Here's how the part is built. I have some questions about the finished solid (model axes, mm). Face numbers are marked on the shaded views. A direction names the side the tool comes from. Round coordinates to 2 decimals unless told otherwise and drop trailing zeros. Write each loop counter-clockwise with the first axis right and the second up, starting at its lowest first coordinate (ties: lowest second). Pieces come first, ordered by that corner, then holes. Notation, with made-up numbers: (-38.75, 59.5) - (-5.75, 59.5) arc R26 cw to (-5.75, 78.5) - close; hole circle Ø2 at (33.25, 30). An arc over 180 degrees is marked (long way). Return JSON: item names as keys, results as strings. Group by question number.
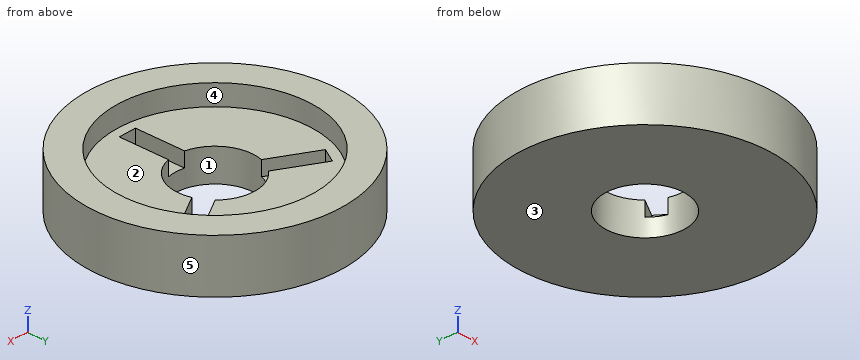
```python
from build123d import *

# Parameters (mm, degrees)
SKETCH_R           = 43.25
PAD_DEPTH          = 18
SKETCH001_R        = 33.25
POCKET_DEPTH       = 7
SKETCH002_R        = 13.5
POCKET001_DEPTH    = 11.001
SKETCH003_W        = 6
SKETCH003_H        = 30
POCKET002_DEPTH    = 5
POLARPATTERN_COUNT = 3


with BuildPart() as part:
    # Sketch → Pad (new body)
    with BuildSketch(Plane.XY):
        Circle(SKETCH_R)
    extrude(amount=PAD_DEPTH)

    # Sketch001 (on Face3 of Pad) → Pocket (cut)
    with BuildSketch(Plane.XY.offset(18)):
        Circle(SKETCH001_R)
    extrude(amount=-POCKET_DEPTH, mode=Mode.SUBTRACT)

    # Sketch002 (on Face5 of Pocket) → Pocket001 (cut, through all)
    with BuildSketch(Plane.XY.offset(11)):
        Circle(SKETCH002_R)
    extrude(amount=-POCKET001_DEPTH, mode=Mode.SUBTRACT)

    # Sketch003 (on Face6 of Pocket001) → Pocket002 (cut)
    with BuildSketch(Plane.XY.offset(11)):
        with Locations((0, -15)):
            Rectangle(SKETCH003_W, SKETCH003_H)
    pocket002 = extrude(amount=-POCKET002_DEPTH, mode=Mode.SUBTRACT)

    # PolarPattern: Pocket002 ×3 about axis
    polarpattern_axis = Axis((0, 0, 11), (0, 0, 1))
    for i in range(1, POLARPATTERN_COUNT):
        add(pocket002.rotate(polarpattern_axis, i * 360 / POLARPATTERN_COUNT), mode=Mode.SUBTRACT)


solid = part.part
```
1) Imagine slicing it at D-D (z = 4.5). Please give me the cut outline in (x, y), plus the area to 3 significant figures.
2) I need wall thicknesses on line 1 along Y through (x, z) = (0, 13.5); line 2 along Y through (x, z) = (0, 3.25); line 3 along X through (y, z) = (1.5, 14.75). Which ranges of each line are inside material? Lowest first, please.
3) Imagine slicing it at A-A (y = 0). Please give me the cut outline in (x, z).
4) For the marked faces 1 and 2, which set-ups out of +Z, -Z, +X, -X, +Y, -Y let a thin tool reach every point of the face, with its end or its side?
5) Imagine slicing it at B-B (x = 0). Please give me the cut outline in (y, z).
6) Imagine slicing it at C-C (x = -30). Please give me the cut outline in (y, z), plus the area to 3 significant figures.
7) If we mould it in two halves opening along Y, with no side actions, what happens to the marked faces 3, 4 and 5? For each: released by +Y, released by -Y, zero draft, split by the parting line, or undercut.
8) Will these pins go through, and if not, where does the flat tip stop? pin 1 Ø10 at (y, z) = (26, 14) entering from -X; pin 2 Ø8 at (x, z) = (-5, 12) entering from -Y; pin 3 Ø4 at (y, z) = (-22, 8.5) entering from -X.
Results found:
{
 "1": {"outline": "circle Ø86.5 at (0, 0); hole circle Ø27 at (0, 0)", "area": "5,300 mm²"},
 "2": {"line 1": "y = -43.25 to -33.25, 33.25 to 43.25", "line 2": "y = -43.25 to -13.5, 13.5 to 43.25", "line 3": "x = -43.22 to -33.22, 33.22 to 43.22"},
 "3": {"outline": "(-43.25, 0) - (-13.5, 0) - (-13.5, 11) - (-33.25, 11) - (-33.25, 18) - (-43.25, 18) - close; (13.5, 0) - (43.25, 0) - (43.25, 18) - (33.25, 18) - (33.25, 11) - (13.5, 11) - close"},
 "4": {"face 1": "+Z, -Z", "face 2": "+Z"},
 "5": {"outline": "(-43.25, 0) - (-13.5, 0) - (-13.5, 6) - (-30, 6) - (-30, 11) - (-33.25, 11) - (-33.25, 18) - (-43.25, 18) - close; (13.5, 0) - (43.25, 0) - (43.25, 18) - (33.25, 18) - (33.25, 11) - (13.5, 11) - close"},
 "6": {"outline": "(-31.15, 0) - (31.15, 0) - (31.15, 18) - (14.34, 18) - (14.34, 11) - (-14.34, 11) - (-14.34, 18) - (-31.15, 18) - close", "area": "921 mm²"},
 "7": {"face 3": "zero draft", "face 4": "undercut", "face 5": "split by the parting line"},
 "8": {"pin 1": "stops at x = -37.81", "pin 2": "stops at y = -43.24", "pin 3": "stops at x = -38.35"}
}
